Can you work these out from the model? Positions are in its coordinate system, mm. A direction names the side the tool comes from. Give positions to 0.01 mm unless a question says otherwise; leave off trailing zeros. Order: outer loops, then holes, each group sorted by start corner. A loop starts at its lowest first (then second) coordinate and runs counter-clockwise, first axis right, second up. Notation, with made-up numbers: M -6.5,61 L 20.5,61 A17 cw 20.5,75 Z; hole C 45.5,13 d5. An arc over 180 degrees is marked long. Write each question's results on one line, items separated by ' | '.
from build123d import *
from OCP.BRepFilletAPI import BRepFilletAPI_MakeChamfer

# Parameters (mm, degrees)
SKETCH1_W           = 224
SKETCH1_H           = 144
BOSS_EXTRUDE1_DEPTH = 42
SKETCH2_W           = 175
SKETCH2_H           = 11
BOSS_EXTRUDE2_DEPTH = 4.5
CHAMFER1_SIZE       = 8.5
CHAMFER1_SIZE2      = 26.5
CHAMFER2_SIZE       = 26.5
CHAMFER2_SIZE2      = 8.5


with BuildPart() as part:
    # Sketch1 → Boss-Extrude1 (new body)
    with BuildSketch(Plane(origin=(0, 0, 0), x_dir=(1, 0, 0), z_dir=(0, 1, 0))):
        with Locations((112, 72)):
            Rectangle(SKETCH1_W, SKETCH1_H)
    extrude(amount=BOSS_EXTRUDE1_DEPTH)

    # Sketch2 → Boss-Extrude2 (add)
    with BuildSketch(Plane.XZ):
        with Locations((112, -128.25)):
            Rectangle(SKETCH2_W, SKETCH2_H)
        with Locations((112, -15.75)):
            Rectangle(SKETCH2_W, SKETCH2_H)
    extrude(amount=BOSS_EXTRUDE2_DEPTH)

    # Chamfer1: one chamfer whose edges measure the first distance from different faces: ONE call of the kernel's chamfer builder (chamfer() names one face for all edges)
    chamfer1_edges_1 = [part.edges().sort_by_distance(p)[0] for p in [
        (224, 21, -144),
    ]]
    chamfer1_side_1 = [part.faces().sort_by_distance(p)[0] for p in [
        (224, 21, -72),
    ]]
    chamfer1_edges_2 = [part.edges().sort_by_distance(p)[0] for p in [
        (0, 21, 0),
    ]]
    chamfer1_side_2 = [part.faces().sort_by_distance(p)[0] for p in [
        (0, 21, -72),
    ]]
    chamfer1 = BRepFilletAPI_MakeChamfer(part.part.solid().wrapped)
    for e in chamfer1_edges_1:
        chamfer1.Add(CHAMFER1_SIZE, CHAMFER1_SIZE2, e.wrapped, chamfer1_side_1[0].wrapped)  # the first distance lies on this face
    for e in chamfer1_edges_2:
        chamfer1.Add(CHAMFER1_SIZE, CHAMFER1_SIZE2, e.wrapped, chamfer1_side_2[0].wrapped)  # the first distance lies on this face
    add(Compound.cast(chamfer1.Shape()), mode=Mode.REPLACE)

    # Chamfer2: one chamfer whose edges measure the first distance from different faces: ONE call of the kernel's chamfer builder (chamfer() names one face for all edges)
    chamfer2_edges_1 = [part.edges().sort_by_distance(p)[0] for p in [
        (0, 21, -144),
    ]]
    chamfer2_side_1 = [part.faces().sort_by_distance(p)[0] for p in [
        (98.75, 21, -144),
    ]]
    chamfer2_edges_2 = [part.edges().sort_by_distance(p)[0] for p in [
        (224, 21, 0),
    ]]
    chamfer2_side_2 = [part.faces().sort_by_distance(p)[0] for p in [
        (125.25, 21, 0),
    ]]
    chamfer2 = BRepFilletAPI_MakeChamfer(part.part.solid().wrapped)
    for e in chamfer2_edges_1:
        chamfer2.Add(CHAMFER2_SIZE, CHAMFER2_SIZE2, e.wrapped, chamfer2_side_1[0].wrapped)  # the first distance lies on this face
    for e in chamfer2_edges_2:
        chamfer2.Add(CHAMFER2_SIZE, CHAMFER2_SIZE2, e.wrapped, chamfer2_side_2[0].wrapped)  # the first distance lies on this face
    add(Compound.cast(chamfer2.Shape()), mode=Mode.REPLACE)


solid = part.part
(1) We'd pull the mould along Z, two halves only. Please class faces 5 (the face through (111, -2, -122.75)), 6 (the face through (210.9, 20.7, -4.3)), 7 (the face through (110, 0, -73)), 8 (the face through (24.5, -2, -128)): +Z half, -Z half, draft (parallel to the pull), parting line (faces both ways), or undercut.
Data:
face 5: undercut | face 6: +Z half | face 7: undercut | face 8: draft
(2) Imagine slicing it at A-A, the plane x = 168. Write out the boundary of the cut face in (y, z).
Data:
outline: M -4.5,-133.75 L 0,-133.75 L 0,-144 L 42,-144 L 42,0 L 0,0 L 0,-10.25 L -4.5,-10.25 L -4.5,-21.25 L 0,-21.25 L 0,-122.75 L -4.5,-122.75 Z
(3) For faces 1 (the face through (111, -2, -10.25)), 2 (the face through (111, -2, -133.75)), 3 (the face through (24.5, -2, -16)), 4 (the face through (199.5, -2, -128)), which set-ups out of +Z, -Z, +X, -X, +Y, -Y let a thin tool reach every point of the face, with its end or its side?
Data:
face 1: +Z, +X, -X, -Y | face 2: -Z, +X, -X, -Y | face 3: +Z, -Z, -X, -Y | face 4: +Z, -Z, +X, -Y
(4) Will these pins go through, and if not, where does the flat tip stop? P1, Ø2, axis at y = -3, z = -15.5, coming from the -X side; P2, Ø1.3, axis at x = 111, y = -2, coming from the +Z side; P3, Ø5, axis at x = 115.5, y = -3.5, coming from the -Z side.
Data:
P1: stops at x = 24.5 | P2: stops at z = -10.25 | P3: stops at z = -133.75
(5) Imagine slicing it at B-B, the plane z = -130.5. Write out the boundary of the cut face in (x, y).
Data:
outline: M 0,0 L 24.5,0 L 24.5,-4.5 L 199.5,-4.5 L 199.5,0 L 224,0 L 224,42 L 0,42 Z
(6) I need wall thicknesses on L1, parallel to Y at x = 209, z = -105; L2, parallel to Z at x = 205, y = 6. Which ranges of each line are inside material? Lowest first, please. Write a range as from..to.
Data:
L1: y = 0..42 | L2: z = -141.59..-2.41
(7) Imagine slicing it at C-C, the plane z = -27. Write out the boundary of the cut face in (x, y), plus the area to 3 significant figures.
Data:
outline: M 0,0 L 224,0 L 224,42 L 0,42 Z | area: 9,410 mm2
(8) Imagine slicing it at D-D, the plane x = 14.5. Write out the boundary of the cut face in (y, z).
Data:
outline: M 0,-140.15 L 42,-140.15 L 42,-3.85 L 0,-3.85 Z
